Here's how the part is built. I have some questions about the finished solid (model axes, mm). Face numbers are marked on the shaded views. A direction names the side the tool comes from. Round coordinates to 2 decimals unless told otherwise and drop trailing zeros. Order: outer loops, then holes, each group sorted by start corner. A loop starts at its lowest first (then second) coordinate and runs counter-clockwise, first axis right, second up. Notation, with made-up numbers: (76, 89) -> (117, 89) arc R11 cw to (117, 106) -> close; hole circle Ø11 at (-28, 80). An arc over 180 degrees is marked (long way). One line per item, written item: value.
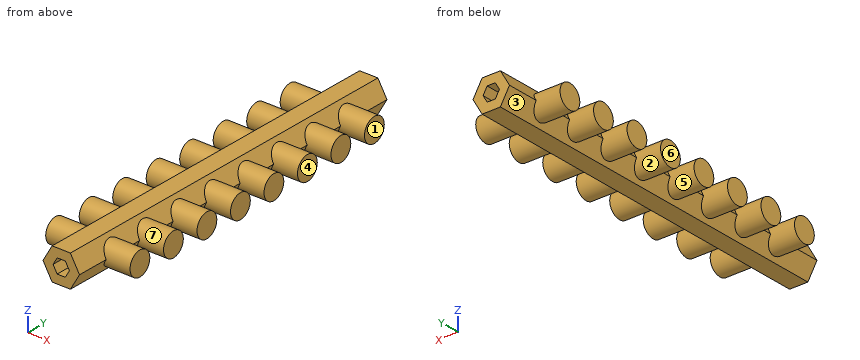
Autodesk Inventor part; units mm, degrees
ref_plane "YZ Plane" through (0, 0, 0) normal (1, 0, 0) x (0, 1, 0)
ref_plane "XZ Plane" through (0, 0, 0) normal (0, 1, 0) x (-1, 0, 0)
ref_plane "XY Plane" through (0, 0, 0) normal (0, 0, 1) x (1, 0, 0)
sketch "Outer Diameter Sketch" plane through (0, 0, 0) normal (0, 1, 0) x (-1, 0, 0)
  line L0 (0, -28.0163) -> (0, 28.3344) construction
  line L1 (17.1062, 0) -> (-23.8822, 0) construction
  line L2 (3.4641, -6) -> (6.9282, 0)
  line L3 (6.9282, 0) -> (3.4641, 6)
  line L4 (3.4641, 6) -> (-3.4641, 6)
  line L5 (-3.4641, 6) -> (-6.9282, 0)
  line L6 (-6.9282, 0) -> (-3.4641, -6)
  line L7 (-3.4641, -6) -> (3.4641, -6)
  line L8 (0, -6) -> (0, 6) construction
  line L9 (-6.9282, 0) -> (6.9282, 0) construction
  point P0 (0, 0)
  dimension "d23" = 120
  dimension "d25" = 120
  dimension "d27" = 120
  dimension "d29" = 120
  dimension "d31" = 120
  dimension "d32" = 12
extrude "Outer Diameter Extrusion" add sketch "Outer Diameter Sketch" along normal mid plane 140
sketch "Sketch2" plane through (0, 0, 0) normal (1, 0, 0) x (0, 1, 0)
  circle A0 centre (-7.625, 0) radius 4.5
  line L0 (-77.625, 0) -> (-7.625, 0) construction
  line L1 (-7.625, 0) -> (62.375, 0) construction
  circle A1 centre (7.625, 0) radius 4.5
  circle A2 centre (22.875, 0) radius 4.5
  circle A3 centre (38.125, 0) radius 4.5
  circle A4 centre (-22.875, 0) radius 4.5
  circle A5 centre (-7.625, 0) radius 4.5
  circle A6 centre (7.625, 0) radius 4.5
  circle A7 centre (22.875, 0) radius 4.5
  circle A8 centre (-38.125, 0) radius 4.5
  circle A9 centre (-22.875, 0) radius 4.5
  circle A10 centre (-7.625, 0) radius 4.5
  circle A11 centre (7.625, 0) radius 4.5
  circle A12 centre (-53.375, 0) radius 4.5
  circle A13 centre (-38.125, 0) radius 4.5
  circle A14 centre (-22.875, 0) radius 4.5
  circle A15 centre (-7.625, 0) radius 4.5
  line L2 (0, 54.0285) -> (0, -72.3739) construction
  circle A16 centre (53.375, 0) radius 4.5
  circle A17 centre (38.125, 0) radius 4.5
  circle A18 centre (22.875, 0) radius 4.5
  circle A19 centre (7.625, 0) radius 4.5
  dimension "d3" = 9
  dimension "d5" = 140
  dimension "d8" = 15.25
  dimension "d11" = 15.25
  dimension "d47" = 7.625
  dimension "d48" = 7.625
extrude "Extrusion2" add sketch "Sketch2" along normal mid plane 32
sketch "Sketch3" plane through (0, -70, 0) normal (0, -1, 0) x (1, 0, 0)
  line L0 (1.55, -2.6847) -> (-1.55, -2.6847)
  line L1 (-1.55, -2.6847) -> (-3.1, 0)
  line L2 (-3.1, 0) -> (-1.55, 2.6847)
  line L3 (-1.55, 2.6847) -> (1.55, 2.6847)
  line L4 (1.55, 2.6847) -> (3.1, 0)
  line L5 (3.1, 0) -> (1.55, -2.6847)
  line L6 (3.1, 0) -> (-3.1, 0) construction
  line L7 (0, 2.6847) -> (0, -2.6847) construction
  line L8 (10.3659, 0) -> (-11.745, 0) construction
  line L9 (0, -9.4896) -> (0, 9.303) construction
  point P0 (0, 0)
  dimension "d33" = 3.1
  dimension "d34" = 3.1
  dimension "d35" = 120
  dimension "d36" = 3.1
  dimension "d37" = 120
  dimension "d38" = 3.1
  dimension "d39" = 120
  dimension "d40" = 3.1
  dimension "d41" = 120
extrude "Extrusion3" cut sketch "Sketch3" against normal up to surface (140 mm away)
equation "\"d1\" = outL"
equation "\"d3\" = pegD"
equation "\"d5\" = outL"
equation "\"d47\" = 0.5 * d8"
equation "\"d14\" = pegL + 2 * outD"
equation "\"d33\" = inhexSL"
equation "\"d34\" = inhexSL"
equation "\"d36\" = inhexSL"
equation "\"d38\" = inhexSL"
equation "\"d40\" = inhexSL"
equation "\"d42\" = pegL + 2 * outD"
equation "\"outD\" = 12"
equation "\"inhexSL\" = 3.1"
equation "\"outL\" = 140"
equation "\"pegL\" = 8"
equation "\"pegD\" = 9"
equation "\"outhexSL\" = 5"
properties part number "Peg Spinner V2"
Q1. I want a section at B-B on x = -8.5. Write out the boundary of the cut face in (y, z) (3 decimals), then the cut area to 3 significant figures.
Answers:
outline: circle Ø9 at (-53.375, 0); circle Ø9 at (-38.125, 0); circle Ø9 at (-22.875, 0); circle Ø9 at (-7.625, 0); circle Ø9 at (7.625, 0); circle Ø9 at (22.875, 0); circle Ø9 at (38.125, 0); circle Ø9 at (53.375, 0)
area: 509 mm2
Q2. I want a section at A-A on y = -14. Write out the boundary of the cut face in (x, z).
Answers:
outline: (-6.93, 0) -> (-3.46, -6) -> (3.46, -6) -> (6.93, 0) -> (3.46, 6) -> (-3.46, 6) -> close; hole (-3.1, 0) -> (-1.55, -2.68) -> (1.55, -2.68) -> (3.1, 0) -> (1.55, 2.68) -> (-1.55, 2.68) -> close
Q3. I need wall thicknesses on line 1 along X through (y, z) = (57, -0.75); line 2 along Z through (x, y) = (-14, -50.5); line 3 along X through (y, z) = (-52, -0.25). Which ranges of each line are inside material? Lowest first, please.
Answers:
line 1: -16 to -2.67, 2.67 to 16
line 2: -3.46 to 3.46
line 3: -16 to -2.96, 2.96 to 16
Q4. I want a section at D-D on y = -53.5. Write out the boundary of the cut face in (x, z), then the cut area to 3 significant figures.
Answers:
outline: (-16, -4.5) -> (-4.33, -4.5) -> (-3.46, -6) -> (3.46, -6) -> (4.33, -4.5) -> (16, -4.5) -> (16, 4.5) -> (4.33, 4.5) -> (3.46, 6) -> (-3.46, 6) -> (-4.33, 4.5) -> (-16, 4.5) -> close; hole (-3.1, 0) -> (-1.55, -2.68) -> (1.55, -2.68) -> (3.1, 0) -> (1.55, 2.68) -> (-1.55, 2.68) -> close
area: 286 mm2
Q5. Which directions (+Z, -Z, +X, -X, +Y, -Y) give clear straight access to the entire face, cutting with the end or side of a thin tool? Please do the marked faces 3, 4, 5, 6 and 7.
Answers:
face 3: -Z, -X
face 4: +Z, -Z, +X, +Y, -Y
face 5: -X
face 6: +Z, -Z, -X, +Y, -Y
face 7: +X
Q6. If we mould it in two halves opening along Y, with no side actions, what happens to the marked faces 1 and 2? For each: pulls with the +Y half, pulls with the -Y half, needs draft (parallel to the pull), parting line crosses it, or undercut.
Answers:
face 1: needs draft
face 2: undercut
Q7. For P1, Ø1, axis at y = 46.5, z = 1.5, coming from the +X side; P2, Ø2, axis at x = 12.5, y = 40.5, coming from the -Z side; P3, Ø1.5, axis at x = 12, z = 0, coming from the -Y side (3 decimals); P4, Ø1, axis at x = 1.5, z = 1.5, coming from the -Y side, each with a flat end and sliding along its axis, tell me the tip position at first contact or that it passes through.
Answers:
P1: x = 6.35
P2: z = -4.28
P3: y = -57.875
P4: through
Q8. I want a section at C-C on y = 39. Write out the boundary of the cut face in (x, z), then the cut area to 3 significant figures.
Answers:
outline: (-16, -4.41) -> (-4.38, -4.41) -> (-3.46, -6) -> (3.46, -6) -> (4.38, -4.41) -> (16, -4.41) -> (16, 4.41) -> (4.38, 4.41) -> (3.46, 6) -> (-3.46, 6) -> (-4.38, 4.41) -> (-16, 4.41) -> close; hole (-3.1, 0) -> (-1.55, -2.68) -> (1.55, -2.68) -> (3.1, 0) -> (1.55, 2.68) -> (-1.55, 2.68) -> close
area: 282 mm2
